For this review, take the finished solid that the model builds, in its own axes (mm). Face numbers are marked on the shaded views. Coordinates: 2 decimals unless noted, no trailing zeros. Order: outer loops, then holes, each group sorted by start corner. A loop starts at its lowest first (then second) coordinate and runs counter-clockwise, first axis right, second up. Notation, with made-up numbers: M 12.25,55.25 L 19.25,55.25 A29 ccw 19.25,77.25 Z; hole C 74.25,3.25 d5. An arc over 180 degrees is marked long. Use CSV: the item, a comma, the result in double quotes.
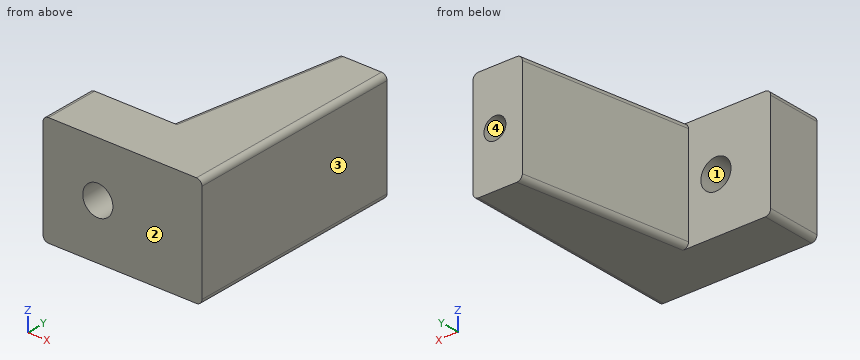
```python
from build123d import *

# Parameters (mm, degrees)
EXTRUDE_1_DEPTH     = 20
SKETCH_2_R          = 2
SKETCH_2_R_2        = 2.75
CUT_EXTRUDE_1_DEPTH = 51.754310162
EXTRUDE_START       = -35
SKETCH_3_R          = 2
EXTRUDE_2_DEPTH     = 35
SKETCH_4_W          = 5
SKETCH_4_H          = 20
EXTRUDE_3_DEPTH     = 10
FILLET_2_R          = 1


with BuildPart() as part:
    # ｽｹｯﾁ1 → ﾎﾞｽ - 押し出し1 (new body)
    with BuildSketch(Plane.XY):
        Polygon((0, 0), (10, 0), (15, 30), (24, 30), (24, -10), (0, -10), align=None)
    extrude(amount=EXTRUDE_1_DEPTH)

    # ｽｹｯﾁ2 → ｶｯﾄ - 押し出し1 (cut, through all)
    with BuildSketch(Plane(origin=(0, 30, 0), x_dir=(1, 0, 0), z_dir=(0, 1, 0))):
        with Locations(Location((20, -10, 0), (0, 0, 270))):
            Circle(SKETCH_2_R)
        with Locations(Location((5, -10, 0), (0, 0, 270))):
            Circle(SKETCH_2_R_2)
    extrude(amount=-CUT_EXTRUDE_1_DEPTH, mode=Mode.SUBTRACT)

    # ｽｹｯﾁ3 → ﾎﾞｽ - 押し出し2 (add)
    with BuildSketch(Plane.XZ.offset(10).offset(EXTRUDE_START)):
        with Locations(Location((20, 10, 0), (0, 0, 90))):
            Circle(SKETCH_3_R)
    extrude(amount=EXTRUDE_2_DEPTH)

    # ｽｹｯﾁ4 → ﾎﾞｽ - 押し出し3 (add)
    with BuildSketch(Plane(origin=(0, 0, 0), x_dir=(1, 0, 0), z_dir=(0, 1, 0))):
        with Locations((-2.5, -10)):
            Rectangle(SKETCH_4_W, SKETCH_4_H)
    extrude(amount=-EXTRUDE_3_DEPTH)

    # ﾌｨﾚｯﾄ2
    fillet_2_edges = [part.edges().sort_by_distance(p)[0] for p in [
        (24, 10, 20),
        (12.5, 15, 20),
        (-5, -5, 20),
        (-5, -5, 0),
        (12.5, 15, 0),
        (24, 10, 0),
    ]]
    fillet(fillet_2_edges, radius=FILLET_2_R)


solid = part.part
```
Item 1: Clearance check with flat-ended pins moving along their axes: pin 1 Ø6 at (x, y) = (7, 14.5) entering from +Z; pin 2 Ø4.5 at (x, z) = (20.5, 9.5) entering from +Y; pin 3 Ø3 at (y, z) = (10, 13.5) entering from -X; pin 4 Ø10 at (y, z) = (15.5, 3.5) entering from -X. State where each tip first meets the part, or that it passes through.
Solutions:
pin 1,"through"
pin 2,"y = 30"
pin 3,"x = 11.42"
pin 4,"x = 11.75"
Item 2: Draft analysis for pull direction X (two halves, no side actions). For the marked faces 1, 2, 3 and 4, state which applies: released by +X, released by -X, zero draft, split by the parting line, or undercut.
Solutions:
face 1,"undercut"
face 2,"zero draft"
face 3,"released by +X"
face 4,"undercut"
Item 3: Add section D-D on x = 20. State the section outline as (y, z) points, and give its area (3 significant figures).
Solutions:
outline,"M -10,0 L 30,0 L 30,8 L 25,8 L 25,12 L 30,12 L 30,20 L -10,20 Z"
area,"780 mm^2"
Item 4: Add section A-A on y = -2. State the section outline as (x, z) points.
Solutions:
outline,"M -5,1 A1 ccw -4,0 L 23,0 A1 ccw 24,1 L 24,19 A1 ccw 23,20 L -4,20 A1 ccw -5,19 Z; hole C 5,10 d5.5"
Item 5: Add section B-B on x = 5. State the section outline as (y, z) points.
Solutions:
outline,"M -10,0 L 0,0 L 0,7.25 L -10,7.25 Z; M -10,12.75 L 0,12.75 L 0,20 L -10,20 Z"
Item 6: To check wall thickness, follow line 1 along X through (y, z) = (-7, 10); line 2 along Z through (x, y) = (20, 28.2); line 3 along X through (y, z) = (26.7, 10). State the ranges of each line that lie inside material, in increasing order. Write a range as [from, to].
Solutions:
line 1,"[-5, 2.25], [7.75, 24]"
line 2,"[0, 8], [12, 20]"
line 3,"[14.45, 18], [22, 24]"
Item 7: Add section C-C on z = 10. State the section outline as (x, y) points, and give its area (3 significant figures).
Solutions:
outline,"M -5,-10 L 2.25,-10 L 2.25,0 L -5,0 Z; M 7.75,-10 L 24,-10 L 24,30 L 22,30 L 22,25 L 18,25 L 18,30 L 15,30 L 10,0 L 7.75,0 Z"
area,"560 mm^2"
